Autodesk Inventor part; units mm, degrees
ref_plane "YZ Plane" through (0, 0, 0) normal (1, 0, 0) x (0, 1, 0)
ref_plane "XZ Plane" through (0, 0, 0) normal (0, 1, 0) x (-1, 0, 0)
ref_plane "XY Plane" through (0, 0, 0) normal (0, 0, 1) x (1, 0, 0)
sketch "Sketch1" plane through (0, 0, 0) normal (0, 1, 0) x (-1, 0, 0)
  line L0 (15, 0) -> (40, 0) construction
  line L1 (-15, 0) -> (-40, 0) construction
  line L2 (14.9248, -1.5) -> (39.9719, -1.5)
  line L3 (14.9248, 1.5) -> (39.9719, 1.5)
  line L4 (-14.9248, -1.5) -> (-39.9719, -1.5)
  line L5 (-14.9248, 1.5) -> (-39.9719, 1.5)
  arc A0 (-39.9719, 1.5) -> (-39.9719, -1.5) centre (0, 0) ccw
  arc A1 (39.9719, -1.5) -> (39.9719, 1.5) centre (0, 0) ccw
  arc A2 (14.9248, 1.5) -> (-14.9248, 1.5) centre (0, 0) ccw
  arc A3 (-14.9248, -1.5) -> (14.9248, -1.5) centre (0, 0) ccw
  dimension "d2" = 1.5
  dimension "d3" = 1.5
  dimension "d4" = 1.5
  dimension "d5" = 1.5
extrude "Extrusion1" add sketch "Sketch1" along normal blind 20
fillet "Fillet1" radius 5 2 edges at (40, 20, 0) (-40, 20, 0)
chamfer "Chamfer1" distance 20 angle 30 1 edges at (-40, 0, 0) measured on face at (-3.3541, 0, 5.1142)
chamfer "Chamfer2" distance 20 angle 30 1 edges at (40, 0, 0) measured on face at (2.3541, 0, 4.4112)
fillet "Fillet2" radius 5 2 edges at (40, 11.547, 0) (-40, 11.547, 0)
fillet "Fillet3" radius 5 2 edges at (20, 0, 0) (-20, 0, 0)
sketch "Sketch3" plane through (0, 20, 0) normal (0, 1, 0) x (1, 0, 0)
  arc A0 (-34.9678, 1.5) -> (-34.9678, -1.5) centre (0, 0) ccw construction
  line L0 (-34.9678, -1.5) -> (-14.9248, -1.5) construction
  arc A1 (-14.9248, -1.5) -> (14.9248, -1.5) centre (0, 0) ccw construction
  line L1 (14.9248, -1.5) -> (34.9678, -1.5) construction
  arc A2 (34.9678, -1.5) -> (34.9678, 1.5) centre (0, 0) ccw construction
  line L2 (34.9678, 1.5) -> (14.9248, 1.5) construction
  arc A3 (14.9248, 1.5) -> (-14.9248, 1.5) centre (0, 0) ccw construction
  line L3 (-14.9248, 1.5) -> (-34.9678, 1.5) construction
  circle A4 centre (0, 0) radius 1.5
  dimension "d36" = 3
extrude "Extrusion2" cut sketch "Sketch3" against normal through all
equation "\"d2\" = 0.5 * blade_width"
equation "\"d3\" = 0.5 * blade_width"
equation "\"d4\" = 0.5 * blade_width"
equation "\"d5\" = 0.5 * blade_width"
equation "\"blade_width\" = 3"
equation "\"d21\" = 0"
equation "\"d22\" = 5"
equation "\"d23\" = 3"
equation "\"d24\" = 5"
equation "\"d25\" = 0"
equation "\"d8\" = 0.5 * blade_width"
equation "\"d9\" = 0.5 * blade_width"
equation "\"d10\" = 0.5 * blade_width"
equation "\"d11\" = 0.5 * blade_width"
equation "\"d12\" = 0.5 * blade_width"
equation "\"d13\" = 0.5 * blade_width"
equation "\"d14\" = 0.5 * blade_width"
equation "\"d15\" = 0.5 * blade_width"
equation "\"d16\" = 0.5 * blade_width"
equation "\"d17\" = 0.5 * blade_width"
equation "\"d18\" = 0.5 * blade_width"
equation "\"d19\" = 0.5 * blade_width"
properties part number "top_propeller"
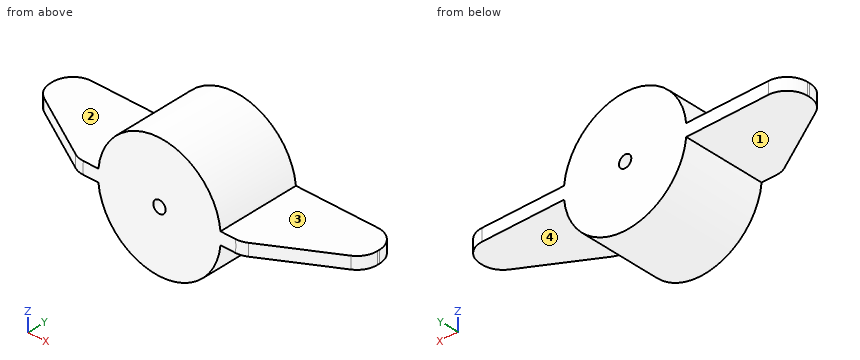
Can you work these out from the model? Positions are in its coordinate system, mm. Face numbers are marked on the shaded views. A direction names the side the tool comes from. Round coordinates to 2 decimals unless told otherwise and drop trailing zeros. Loops run counter-clockwise (first coordinate to the right, second up) from the corner with the lowest first, then second, coordinate; pieces in that order, holes last. Notation, with made-up numbers: M 31.25,-22 L 82.25,-22 A14 cw 82.25,0 Z; hole C 67,41 d3. An arc over 180 degrees is marked long. Write item = value, one per line. Start each with the question number.
(1) I'm going to push flat-ended pins straight in: P1, Ø3, axis at y = 9.5, z = 7.5, coming from the -X side; P2, Ø5, axis at x = -18, y = 15, coming from the -Z side; P3, Ø6, axis at x = -30.5, y = 14.5, coming from the +Z side. Where does each tip first touch, or does it pass through?
(2) Suppose I cut it at A-A on x = 0. Write out the boundary of the cut face in (y, z).
(3) Suppose I cut it at C-C on y = 6. Write out the boundary of the cut face in (x, z), plus the area to 3 significant figures.
(4) Suppose I cut it at D-D on z = -8.25. Write out the boundary of the cut face in (x, y), plus the area to 3 significant figures.
(5) I need wall thicknesses on line 1 along Z through (x, y) = (0, 10.5); line 2 along Z through (x, y) = (28.5, 18); line 3 along X through (y, z) = (6.25, 0). Which ranges of each line are inside material? Lowest first, please.
(6) Suppose I cut it at B-B on y = 18.25. Write out the boundary of the cut face in (x, z), plus the area to 3 significant figures.
(7) Which directions (+Z, -Z, +X, -X, +Y, -Y) give clear straight access to the entire face, cutting with the end or side of a thin tool? Please do the marked faces 1, 2, 3 and 4.
Answer block:
q1.P1 = -13.75
q1.P2 = -1.5
q1.P3 = 1.5
q2.outline = M 0,-15 L 20,-15 L 20,-1.5 L 0,-1.5 Z; M 0,1.5 L 20,1.5 L 20,15 L 0,15 Z
q3.outline = M -30.36,-1.5 L -14.92,-1.5 A15 ccw 14.92,-1.5 L 30.36,-1.5 A30.39 ccw 30.36,1.5 L 14.92,1.5 A15 ccw -14.92,1.5 L -30.36,1.5 A30.39 ccw Z; hole C 0,0 d3
q3.area = 792 mm²
q4.outline = M -12.53,0 L 12.53,0 L 12.53,20 L -12.53,20 Z
q4.area = 501 mm²
q5.line_1 = -15 to -1.5, 1.5 to 15
q5.line_2 = -1.5 to 1.5
q5.line_3 = -30.83 to -1.5, 1.5 to 30.83
q6.outline = M -38.77,-1.5 L -14.92,-1.5 A15 ccw 14.92,-1.5 L 38.77,-1.5 A38.8 ccw 38.77,1.5 L 14.92,1.5 A15 ccw -14.92,1.5 L -38.77,1.5 A38.8 ccw Z; hole C 0,0 d3
q6.area = 843 mm²
q7.face_1 = -Z, -X, +Y, -Y
q7.face_2 = +Z, -X, +Y, -Y
q7.face_3 = +Z, +X, +Y, -Y
q7.face_4 = -Z, +X, +Y, -Y
